```python
from build123d import *

# Parameters (mm, degrees)
F1_DEPTH = 25
F2_R     = 100
F3_DEPTH = 25.001
F4_R     = 78.250027
F5_DEPTH = 164.82871
F7_DEPTH = 189.82971


with BuildPart() as f1:
    # F0 (on Front) → F1 (new body)
    with BuildSketch(Plane.XZ):
        Polygon((-8614.96765, 1097.854802), (-9614.96765, 1097.854802), (-8614.96765, 97.854802), align=None)
    extrude(amount=F1_DEPTH)

    # F2 (on face) → F3 (cut, through all)
    with BuildSketch(Plane.XZ.offset(25)):
        with Locations((-8914.96765, 797.854802)):
            Circle(F2_R)
    extrude(amount=-F3_DEPTH, mode=Mode.SUBTRACT)

    # F4 (on face) → F5 (join)
    with BuildSketch(Plane.XZ.offset(25)):
        with Locations((-9224.896431, 985.964417)):
            Circle(F4_R)
    extrude(amount=F5_DEPTH)

    # F6 (on face) → F7 (cut, through all)
    with BuildSketch(Plane.XZ.offset(189.82871)):
        Polygon((-9229.896431, 977.304163), (-9219.896431, 977.304163), (-9214.896431, 985.964417), (-9219.896431, 994.624671), (-9229.896431, 994.624671), (-9234.896431, 985.964417), align=None)
    extrude(amount=-F7_DEPTH, mode=Mode.SUBTRACT)


solid = f1.part
```
Input: part model. Units: mm. Frame: model coordinates. Give positions to 0.01 mm unless a question says otherwise; leave off trailing zeros. Order: outer loops, then holes, each group sorted by start corner. A loop starts at its lowest first (then second) coordinate and runs counter-clockwise, first axis right, second up.
1. Cut plane D-D (x = -9188). Return loops of the section in (y, z).
Computed:
outline: (-189.83, 916.96) - (-25, 916.96) - (-25, 670.89) - (0, 670.89) - (0, 1097.85) - (-25, 1097.85) - (-25, 1054.97) - (-189.83, 1054.97) - close
2. Line query: probe 1 along Y at (x, z) = (-8809.5, 988); probe 2 along X at (y, z) = (-108.5, 926.5); probe 3 along X at (y, z) = (-81, 968). Output: solid intervals per line, ascending.
Computed:
probe 1: y = -25 to 0
probe 2: x = -9275.76 to -9174.03
probe 3: x = -9301.06 to -9148.74
3. Cut plane A-A (y = -173.5). Return loops of the section in (x, z), and give its area (3 significant figures).
Computed:
outline: circle Ø156.5 at (-9224.9, 985.96); hole (-9234.9, 985.96) - (-9229.9, 977.3) - (-9219.9, 977.3) - (-9214.9, 985.96) - (-9219.9, 994.62) - (-9229.9, 994.62) - close
area: 19,000 mm2
4. Cut plane B-B (z = 737). Return loops of the section in (x, y).
Computed:
outline: (-9254.11, -25) - (-8994.32, -25) - (-8994.32, 0) - (-9254.11, 0) - close; (-8835.62, -25) - (-8614.97, -25) - (-8614.97, 0) - (-8835.62, 0) - close
5. Draft query along X for faces 1 (the face through (-9150.26, -106.26, 1009.47)), 2 (the face through (-9014.87, -12.68, 802.25)), 3 (the face through (-9011, 0, 827)). Return one class per face: released by +X, released by -X, zero draft, split by the parting line, or undercut.
Computed:
face 1: split by the parting line
face 2: undercut
face 3: zero draft
6. Pin query (flat end, axial travel): pin 1 Ø11 at (x, y) = (-9224, -54) entering from +Z; pin 2 Ø12 at (x, z) = (-9358, 953) entering from -Y; pin 3 Ø3 at (x, y) = (-9223, -88) entering from -Z. Return the tip coordinate at first contact, or that it passes through.
Computed:
pin 1: stops at z = 1064.21
pin 2: stops at y = -25
pin 3: stops at z = 907.72
7. Cut plane C-C (x = -8905). Return loops of the section in (y, z), and give its area (3 significant figures).
Computed:
outline: (-25, 387.89) - (0, 387.89) - (0, 698.35) - (-25, 698.35) - close; (-25, 897.36) - (0, 897.36) - (0, 1097.85) - (-25, 1097.85) - close
area: 12,800 mm2
